from build123d import *

# Parameters (mm, degrees)
SKETCH2_R           = 4.191
BOSS_EXTRUDE1_DEPTH = 4.7625
SKETCH4_R           = 5.08
BOSS_EXTRUDE2_DEPTH = 9.8425
BOSS_EXTRUDE2_TAPER = 2
SKETCH6_R           = 4.826
BOSS_EXTRUDE3_DEPTH = 9.8425


with BuildPart() as part:
    # Sweep1: sweep along a path in Sketch1
    with BuildLine(Plane(origin=(0, 0, 0), x_dir=(0, 0, -1), z_dir=(1, 0, 0))) as sweep1_path:
        ThreePointArc((0, 0), (60.651495576, 2.863871037), (120.763284, 11.43))
    # Sketch2 → Sweep1 (sweep)
    with BuildSketch(Plane.XY):
        Circle(SKETCH2_R)
    sweep(path=sweep1_path.line)

    # Sketch3 → Boss-Extrude1 (add)
    with BuildSketch(Plane.XY):
        Polygon((7.332348419, 0), (3.666174209, 6.35), (-3.666174209, 6.35), (-7.332348419, 0), (-3.666174209, -6.35), (3.666174209, -6.35), align=None)
    boss_extrude1 = extrude(amount=BOSS_EXTRUDE1_DEPTH)

    # Sketch4 → Boss-Extrude2 (add)
    with BuildSketch(Plane.XY.offset(4.7625)):
        Circle(SKETCH4_R)
    boss_extrude2 = extrude(amount=BOSS_EXTRUDE2_DEPTH, taper=BOSS_EXTRUDE2_TAPER)

    # Sketch6 → Boss-Extrude3 (add)
    with BuildSketch(Plane(origin=(0, 0, 0), x_dir=(-1, 0, 0), z_dir=(0, 0, -1))):
        with Locations(Location((0, 0, 0), (0, 0, 180))):
            Circle(SKETCH6_R)
    boss_extrude3 = extrude(amount=BOSS_EXTRUDE3_DEPTH)

    # Mirror1: Boss-Extrude1, Boss-Extrude2, Boss-Extrude3 across plane
    add(boss_extrude1.mirror(Plane(origin=(0, 5.715, -60.381642), x_dir=(1, 0, 0), z_dir=(0, 0.09422686028954569, -0.9955507514938526))))
    add(boss_extrude2.mirror(Plane(origin=(0, 5.715, -60.381642), x_dir=(1, 0, 0), z_dir=(0, 0.09422686028954569, -0.9955507514938526))))
    add(boss_extrude3.mirror(Plane(origin=(0, 5.715, -60.381642), x_dir=(1, 0, 0), z_dir=(0, 0.09422686028954569, -0.9955507514938526))))


solid = part.part
Design review of the part built by this model. Coordinates are the model's own, in mm. A direction names the side the tool comes from. Coordinates: 2 decimals unless noted, no trailing zeros. Use one line per item in the form item = value.
(1) Draft analysis for pull direction Z (two halves, no side actions). For faces 4 (the face through (3.77, 8.66, -126.14)), 5 (the face through (-5.525, 8.796, -123.657)), 6 (the face through (5.525, 3.131, 2.348)), state which applies: pulls with the +Z half, pulls with the -Z half, needs draft (parallel to the pull), parting line crosses it, or undercut.
Return value:
face_4 = undercut
face_5 = pulls with the -Z half
face_6 = needs draft
(2) For faces 1 (the face through (-0.051, 5.633, -124.261)), 2 (the face through (0, 6.35, 2)), 3 (the face through (-3.83, 2.937, -4.852)), list the 3-axis set-ups (+Z, -Z, +X, -X, +Y, -Y) from which the entire face can be reached by the end or side of a thin tool; tool diameter is ignored.
Return value:
face_1 = -Z, +X, -X, -Y
face_2 = +Z, +X, -X, +Y
face_3 = none
(3) Clearance check with flat-ended pins moving along their axes: P1, Ø6, axis at x = 3, z = -63, coming from the -Y side; P2, Ø1.4, axis at x = -1, z = 3.5, coming from the +Y side; P3, Ø6, axis at x = -3.5, z = -12.5, coming from the +Y side. State where each tip first meets the part, or that it passes through.
Return value:
P1 = -1.25
P2 = 6.35
P3 = 4.34
(4) For line 1 along Z through (x, y) = (5.5, -2); line 2 along Y through (x, z) = (2.5, 3); line 3 along X through (y, z) = (-1.5, -6.5), list the stretches that pass through material, from the lowest coordinate up. Write a range as from..to.
Return value:
line_1 = 0..4.76
line_2 = -6.35..6.35
line_3 = -4.59..4.59
